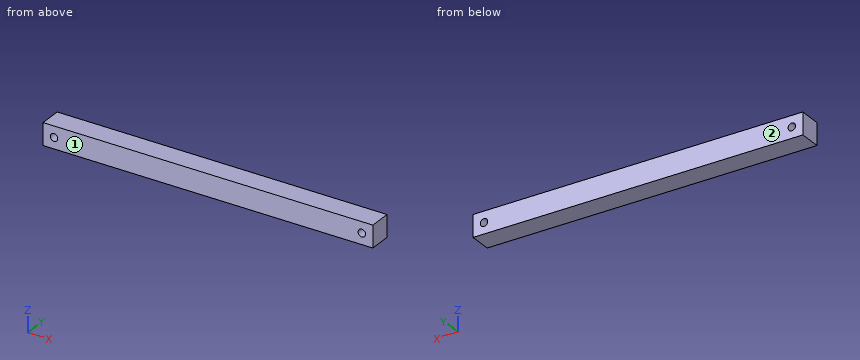
Autodesk Inventor part; units mm, degrees
ref_plane "YZ Plane" through (0, 0, 0) normal (1, 0, 0) x (0, 1, 0)
ref_plane "XZ Plane" through (0, 0, 0) normal (0, 1, 0) x (-1, 0, 0)
ref_plane "XY Plane" through (0, 0, 0) normal (0, 0, 1) x (1, 0, 0)
sketch "スケッチ1" plane through (0, 0, 0) normal (0, 0, 1) x (1, 0, 0)
  line L0 (0, 0) -> (150, 0)
  line L1 (150, 0) -> (150, 10)
  line L2 (150, 10) -> (0, 10)
  line L3 (0, 10) -> (0, 0)
  dimension "d0" = 10
  dimension "d1" = 150
extrude "押し出し1" add sketch "スケッチ1" along normal blind 10
sketch "スケッチ2" plane through (0, 10, 0) normal (0, 1, 0) x (1, 0, 0)
  line L0 (150, 0) -> (0, 0)
  line L1 (0, 0) -> (0, -10)
  line L2 (75, 0) -> (75, -10)
  line L3 (150, -10) -> (0, -10)
  point P0 (5, -5)
  point P1 (145, -5)
  dimension "d4" = 5
  dimension "d5" = 5
hole "穴1" at (5, 10, 5) at (145, 10, 5) direction (0, -1, 0) diameter 3.4 end through all
properties part number "レール"
Design review of the part built by this model. Coordinates are the model's own, in mm. Face numbers are marked on the shaded views. Coordinates: 2 decimals unless noted, no trailing zeros. Order: outer loops, then holes, each group sorted by start corner. A loop starts at its lowest first (then second) coordinate and runs counter-clockwise, first axis right, second up.
Item 1: Take a section at B-B, the plane z = 5. Write out the cut boundary in (x, y), then the cut area to 3 significant figures.
Item 2: For line 1 (X direction, y = 9.25, z = 4.75); line 2 (Z direction, x = 5, y = 4.5); line 3 (X direction, y = 5, z = 6.25), list the stretches that pass through material, from the lowest coordinate up.
Item 3: Take a section at A-A, the plane x = 145. Write out the cut boundary in (y, z).
Item 4: The part is to be moulded in two halves that separate along Y. For the marked faces 1 and 2, say which applies: pulls with the +Y half, pulls with the -Y half, needs draft (parallel to the pull), parting line crosses it, or undercut.
The answers:
1. outline: (0, 0) - (3.3, 0) - (3.3, 10) - (0, 10) - close; (6.7, 0) - (143.3, 0) - (143.3, 10) - (6.7, 10) - close; (146.7, 0) - (150, 0) - (150, 10) - (146.7, 10) - close
1. area: 1,430 mm2
2. line 1: x = 0 to 3.32, 6.68 to 143.32, 146.68 to 150
2. line 2: z = 0 to 3.3, 6.7 to 10
2. line 3: x = 0 to 3.85, 6.15 to 143.85, 146.15 to 150
3. outline: (0, 0) - (10, 0) - (10, 3.3) - (0, 3.3) - close; (0, 6.7) - (10, 6.7) - (10, 10) - (0, 10) - close
4. face 1: pulls with the -Y half
4. face 2: pulls with the +Y half
